Could you check a few things on this model? Use its own coordinates, in mm. Face numbers are marked on the shaded views. A direction names the side the tool comes from. Coordinates: 2 decimals unless noted, no trailing zeros. Write each loop counter-clockwise with the first axis right and the second up, starting at its lowest first coordinate (ties: lowest second). Pieces come first, ordered by that corner, then holes.
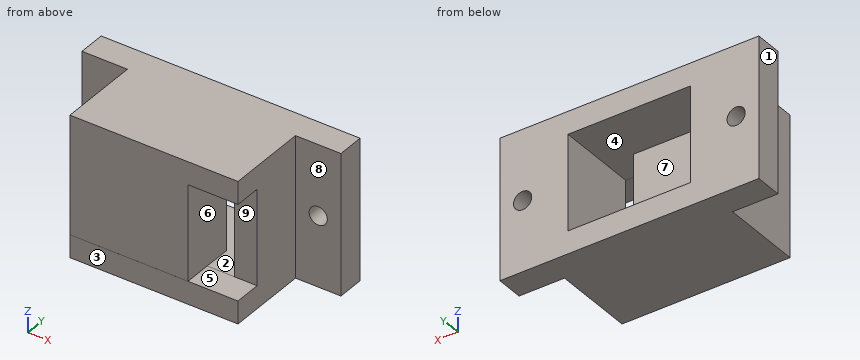
```python
from build123d import *

# Parameters (mm, degrees)
SKETCH2_W           = 18.5
SKETCH2_H           = 15.5
BOSS_EXTRUDE1_DEPTH = 11
SKETCH3_W           = 18.5
SKETCH3_H           = 15.5
BOSS_EXTRUDE2_DEPTH = 3
SKETCH4_W           = 13.5
SKETCH4_H           = 10.5
CUT_EXTRUDE1_DEPTH  = 6
SKETCH5_W           = 3
SKETCH5_H           = 10.5
CUT_EXTRUDE2_DEPTH  = 26
SKETCH10_W          = 18.5
SKETCH10_H          = 5
CUT_EXTRUDE3_DEPTH  = 26
SKETCH11_W          = 15.5
SKETCH11_H          = 3
BOSS_EXTRUDE3_DEPTH = 5
SKETCH13_W          = 18.5
SKETCH13_H          = 2.498768597
BOSS_EXTRUDE4_DEPTH = 3
SKETCH14_W          = 15.5
SKETCH14_H          = 3
BOSS_EXTRUDE6_DEPTH = 5
SKETCH16_R          = 1
CUT_EXTRUDE5_DEPTH  = 5


with BuildPart() as part:
    # Sketch2 → Boss-Extrude1 (new body)
    with BuildSketch(Plane(origin=(0, 0, 0), x_dir=(1, 0, 0), z_dir=(0, 1, 0))):
        with Locations((-3.622916667, -0.966666667)):
            Rectangle(SKETCH2_W, SKETCH2_H)
    extrude(amount=BOSS_EXTRUDE1_DEPTH)

    # Sketch3 → Boss-Extrude2 (add)
    with BuildSketch(Plane(origin=(0, 11, 0), x_dir=(1, 0, 0), z_dir=(0, 1, 0))):
        with Locations((-3.622916667, -0.966666667)):
            Rectangle(SKETCH3_W, SKETCH3_H)
    extrude(amount=BOSS_EXTRUDE2_DEPTH)

    # Sketch4 → Cut-Extrude1 (cut)
    with BuildSketch(Plane(origin=(0, 14, 0), x_dir=(1, 0, 0), z_dir=(0, 1, 0))):
        with Locations((-3.622916667, -0.966666667)):
            Rectangle(SKETCH4_W, SKETCH4_H)
    extrude(amount=-CUT_EXTRUDE1_DEPTH, mode=Mode.SUBTRACT)

    # Sketch5 → Cut-Extrude2 (cut)
    with BuildSketch(Plane(origin=(0, 8, 0), x_dir=(1, 0, 0), z_dir=(0, 1, 0))):
        with Locations((1.627083333, -0.966666667)):
            Rectangle(SKETCH5_W, SKETCH5_H)
    extrude(amount=-CUT_EXTRUDE2_DEPTH, mode=Mode.SUBTRACT)

    # Sketch10 → Cut-Extrude3 (cut)
    with BuildSketch(Plane.XY.offset(8.716666667)):
        with Locations((-3.622916667, 2.5)):
            Rectangle(SKETCH10_W, SKETCH10_H)
    extrude(amount=-CUT_EXTRUDE3_DEPTH, mode=Mode.SUBTRACT)

    # Sketch11 → Boss-Extrude3 (add)
    with BuildSketch(Plane(origin=(5.627083333, 0, 0), x_dir=(0, 0, -1), z_dir=(1, 0, 0))):
        with Locations((-0.966666667, 12.5)):
            Rectangle(SKETCH11_W, SKETCH11_H)
    extrude(amount=BOSS_EXTRUDE3_DEPTH)

    # Sketch13 → Boss-Extrude4 (add)
    with BuildSketch(Plane.XZ.offset(-5)):
        Polygon((5.627083333, 6.217898069), (5.627083333, 8.716666667), (-12.872916667, 8.716666667), (-12.872916667, 6.217898069), (0.127083333, 6.217898069), align=None)
        Polygon((0.127083333, 6.217898069), (-12.872916667, 6.217898069), (-12.872916667, -4.283333333), (0.127083333, -4.283333333), (0.127083333, 6.216666667), align=None)
        with Locations((-3.622916667, -5.533949035)):
            Rectangle(SKETCH13_W, SKETCH13_H)
    extrude(amount=BOSS_EXTRUDE4_DEPTH)

    # Sketch14 → Boss-Extrude6 (add)
    with BuildSketch(Plane.ZY.offset(12.872916667)):
        with Locations((0.966666667, 12.5)):
            Rectangle(SKETCH14_W, SKETCH14_H)
    extrude(amount=BOSS_EXTRUDE6_DEPTH)

    # Sketch16 → Cut-Extrude5 (cut)
    with BuildSketch(Plane(origin=(0, 14, 0), x_dir=(1, 0, 0), z_dir=(0, 1, 0))):
        with Locations(Location((-15.372916667, -0.966666667, 0), (0, 0, 270))):
            Circle(SKETCH16_R)
        with Locations(Location((8.127083333, -0.966666667, 0), (0, 0, 270))):
            Circle(SKETCH16_R)
    extrude(amount=-CUT_EXTRUDE5_DEPTH, mode=Mode.SUBTRACT)


solid = part.part
```
1. For pin 1 (1.8 mm diameter, centred on x = 8.13, z = 0.97, fed in from -Y); pin 2 (8 mm diameter, centred on x = -3.5, z = -1.5, fed in from +Y); pin 3 (4 mm diameter, centred on x = 7.5, z = 3, fed in from -Y); pin 4 (6 mm diameter, centred on y = 5, z = 1, fed in from +X), each with a flat end and sliding along its axis, tell me the tip position at first contact or that it passes through.
Verdict:
pin 1: passes through
pin 2: stops at y = 14
pin 3: stops at y = 5
pin 4: stops at x = 5.63
2. I want a section at A-A on y = 10.5. Please give me the cut outline in (x, z).
Verdict:
outline: (-12.87, -6.78) - (5.63, -6.78) - (5.63, 8.72) - (-12.87, 8.72) - close; hole (-10.37, -4.28) - (3.13, -4.28) - (3.13, 6.22) - (-10.37, 6.22) - close
3. On a 3-axis mill with a long thin cutter (end or side, diameter ignored), from which of +Z, -Z, +X, -X, +Y, -Y can I reach the whole of each face in a straight line? I mean the marked faces 5, 6, 7, 8 and 9. Say none if no direction works.
Verdict:
face 5: none
face 6: +Y, -Y
face 7: +Y
face 8: +Z, -Z, +X, -Y
face 9: +X, -Y
4. Please list where these lines run through material, in increasing order: line 1 along X through (y, z) = (6.75, 3.25); line 2 along Z through (x, y) = (-1, 9.5); line 3 along X through (y, z) = (8.5, 0.25).
Verdict:
line 1: x = -12.87 to 0.13, 3.13 to 5.63
line 2: z = -6.78 to -4.28, 6.22 to 8.72
line 3: x = -12.87 to -10.37, 3.13 to 5.63
5. I want a section at D-D on z = 1.25. Please give me the cut outline in (x, y), plus the area to 3 significant figures.
Verdict:
outline: (-17.87, 11) - (-16.33, 11) - (-16.33, 14) - (-17.87, 14) - close; (-14.41, 11) - (-12.87, 11) - (-12.87, 2) - (0.13, 2) - (0.13, 8) - (-10.37, 8) - (-10.37, 14) - (-14.41, 14) - close; (3.13, 5) - (5.63, 5) - (5.63, 11) - (7.17, 11) - (7.17, 14) - (3.13, 14) - close; (9.09, 11) - (10.63, 11) - (10.63, 14) - (9.09, 14) - close
area: 134 mm2
6. I want a section at B-B on z = 3.5. Please give me the cut outline in (x, y).
Verdict:
outline: (-17.87, 11) - (-12.87, 11) - (-12.87, 2) - (0.13, 2) - (0.13, 8) - (-10.37, 8) - (-10.37, 14) - (-17.87, 14) - close; (3.13, 5) - (5.63, 5) - (5.63, 11) - (10.63, 11) - (10.63, 14) - (3.13, 14) - close
7. If we mould it in two halves opening along X, with no side actions, what happens to the marked faces 1, 2, 3 and 4? For each: pulls with the +X half, pulls with the -X half, needs draft (parallel to the pull), parting line crosses it, or undercut.
Verdict:
face 1: pulls with the -X half
face 2: undercut
face 3: needs draft
face 4: undercut
